Geometry check sheet. Reference: the model listing, model coordinates, mm. Coordinates: 2 decimals unless noted, no trailing zeros. Use a Markdown table: item, result.
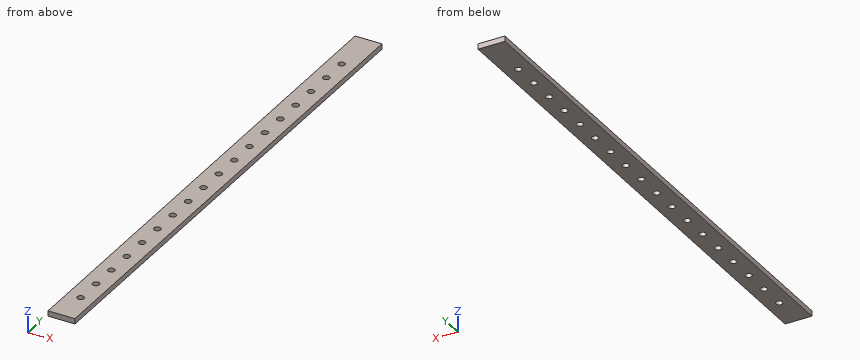
```python
from build123d import *

# Parameters (mm, degrees)
SKETCH_1_W          = 20
SKETCH_1_H          = 4
EXTRUDE_1_DEPTH     = 400
SKETCH_2_R          = 2.5
CUT_EXTRUDE_1_DEPTH = 5


with BuildPart() as part:
    # Эскиз1 → Бобышка-Вытянуть1 (new body)
    with BuildSketch(Plane(origin=(0, 0, 0), x_dir=(1, 0, 0), z_dir=(0, 1, 0))):
        Rectangle(SKETCH_1_W, SKETCH_1_H)
    extrude(amount=EXTRUDE_1_DEPTH)

    # Эскиз2 → Вырез-Вытянуть1 (cut, through all)
    with BuildSketch(Plane.XY.offset(2)):
        with Locations((0, 25)):
            Circle(SKETCH_2_R)
        with Locations((0, 45)):
            Circle(SKETCH_2_R)
        with Locations((0, 65)):
            Circle(SKETCH_2_R)
        with Locations((0, 85)):
            Circle(SKETCH_2_R)
        with Locations((0, 105)):
            Circle(SKETCH_2_R)
        with Locations((0, 125)):
            Circle(SKETCH_2_R)
        with Locations((0, 145)):
            Circle(SKETCH_2_R)
        with Locations((0, 165)):
            Circle(SKETCH_2_R)
        with Locations((0, 185)):
            Circle(SKETCH_2_R)
        with Locations((0, 205)):
            Circle(SKETCH_2_R)
        with Locations((0, 225)):
            Circle(SKETCH_2_R)
        with Locations((0, 245)):
            Circle(SKETCH_2_R)
        with Locations((0, 265)):
            Circle(SKETCH_2_R)
        with Locations((0, 285)):
            Circle(SKETCH_2_R)
        with Locations((0, 305)):
            Circle(SKETCH_2_R)
        with Locations((0, 325)):
            Circle(SKETCH_2_R)
        with Locations((0, 345)):
            Circle(SKETCH_2_R)
        with Locations((0, 365)):
            Circle(SKETCH_2_R)
    extrude(amount=-CUT_EXTRUDE_1_DEPTH, mode=Mode.SUBTRACT)


solid = part.part
```
Item 1: Depth check by flat-ended pin: P1, Ø4.5, axis at x = 0, y = 285, coming from the +Z side; P2, Ø6, axis at x = 0, y = 65, coming from the -Z side. Enter the tip coordinate at first touch or a pass-through.
Answer block:
| item | result |
|---|---|
| P1 | passes through |
| P2 | stops at z = -2 |
Item 2: Section check A-A on z = -0.4. Count the separate pieces of the cut face and the enclosed holes in it, then the cut area to 3 significant figures.
Answer block:
| item | result |
|---|---|
| separate pieces | 1 |
| enclosed holes | 18 |
| area | 7,650 mm^2 |
Item 3: Thickness scan on L1, parallel to X at y = 165, z = 0.15. Record the ranges inside material, lowest first. Write a range as [from, to].
Answer block:
| item | result |
|---|---|
| L1 | x = [-10, -2.5], [2.5, 10] |
